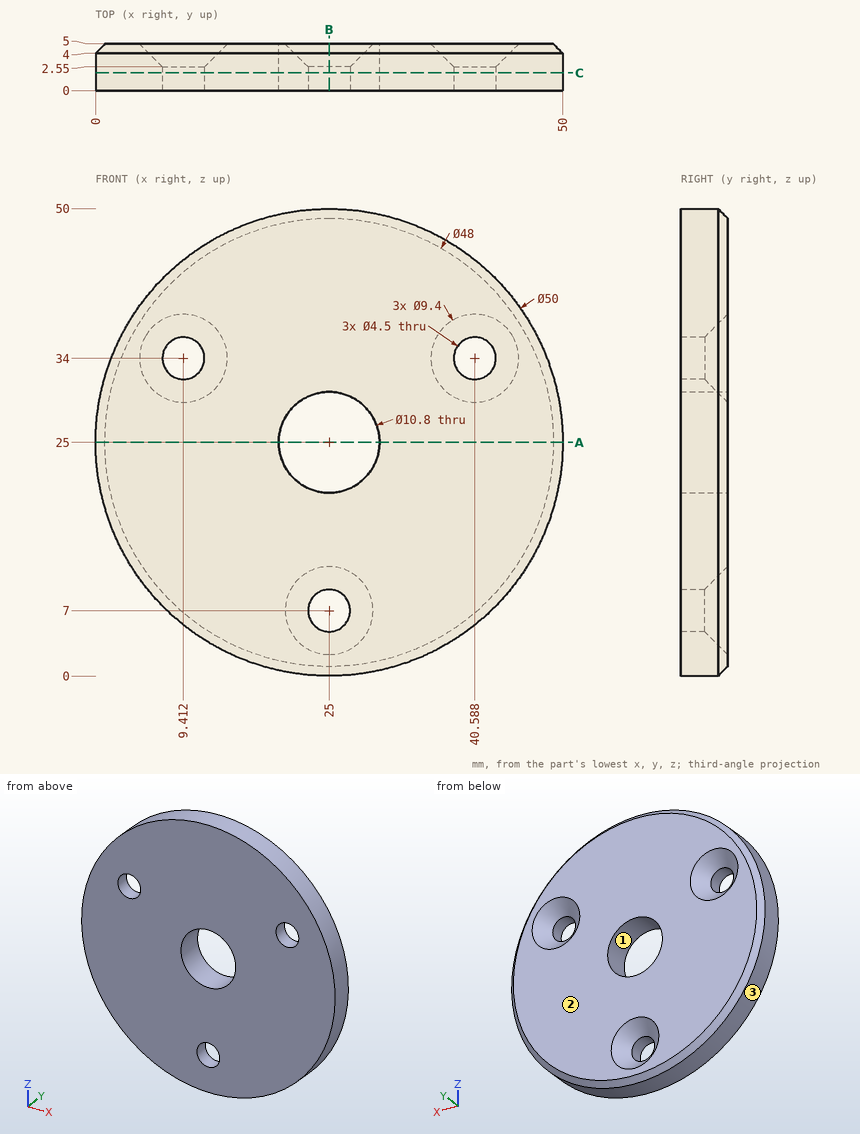
Input: dimensioned drawing with shaded views. Units: mm. Origin: part minimum x, y, z. Coordinates: 2 decimals unless noted, no trailing zeros. Loops run counter-clockwise (first coordinate to the right, second up) from the corner with the lowest first, then second, coordinate; pieces in that order, holes last. Notation, with made-up numbers: (-39, 50) -> (3, 50) arc R32 cw to (3, 88) -> close; hole circle Ø11 at (66, 57.25). An arc over 180 degrees is marked (long way). One line per item, written item: value. Start each with the question number.
Q1. Section query C-C, the plane y = 1.9. Give the number of separate pieces and of enclosed holes in the cut face, and give its area (3 significant figures).
Q2. Mould query, pull axis Z, two halves, no side actions, for the marked faces 1, 2 and 3. Classes: pulls with the +Z half, pulls with the -Z half, needs draft (parallel to the pull), parting line crosses it, or undercut.
Q3. Section query A-A, the plane z = 25. Return the cut outline in (x, y), and give its area (3 significant figures).
Q4. Contact query for flat-ended pins moving along their axis: P1, Ø4, axis at x = 9.41, z = 34, coming from the -Y side; P2, Ø3, axis at y = 2.5, z = 14.5, coming from the +X side; P3, Ø2, axis at y = 1.5, z = 12.5, coming from the +X side; P4, Ø1, axis at x = 14, y = 3, coming from the +Z side. Output: stop coordinate, or through.
Q5. Section query B-B, the plane x = 25. Return the cut outline in (y, z).
Q6. Line query: line 1 along X through (y, z) = (3.05, 25); line 2 along X through (y, z) = (0.9, 34) (1 decimal); line 3 along X through (y, z) = (1.65, 34.5) (1 decimal). Output: solid intervals per line, ascending.
Results:
1. separate pieces: 1
1. enclosed holes: 4
1. area: 1,820 mm^2
2. face 1: undercut
2. face 2: needs draft
2. face 3: parting line crosses it
3. outline: (0, 0) -> (19.6, 0) -> (19.6, 5) -> (1, 5) -> (0, 4) -> close; (30.4, 0) -> (50, 0) -> (50, 4) -> (49, 5) -> (30.4, 5) -> close
3. area: 195 mm^2
4. P1: through
4. P2: x = 48.32
4. P3: x = 47.2
4. P4: z = 47.69
5. outline: (0, 0) -> (4, 0) -> (5, 1) -> (5, 2.3) -> (2.55, 4.75) -> (0, 4.75) -> close; (0, 9.25) -> (2.55, 9.25) -> (5, 11.7) -> (5, 19.6) -> (0, 19.6) -> close; (0, 30.4) -> (5, 30.4) -> (5, 49) -> (4, 50) -> (0, 50) -> close
6. line 1: 0 to 19.6, 30.4 to 50
6. line 2: 1.7 to 7.2, 11.7 to 38.3, 42.8 to 48.3
6. line 3: 1.9 to 7.2, 11.6 to 38.4, 42.8 to 48.1
